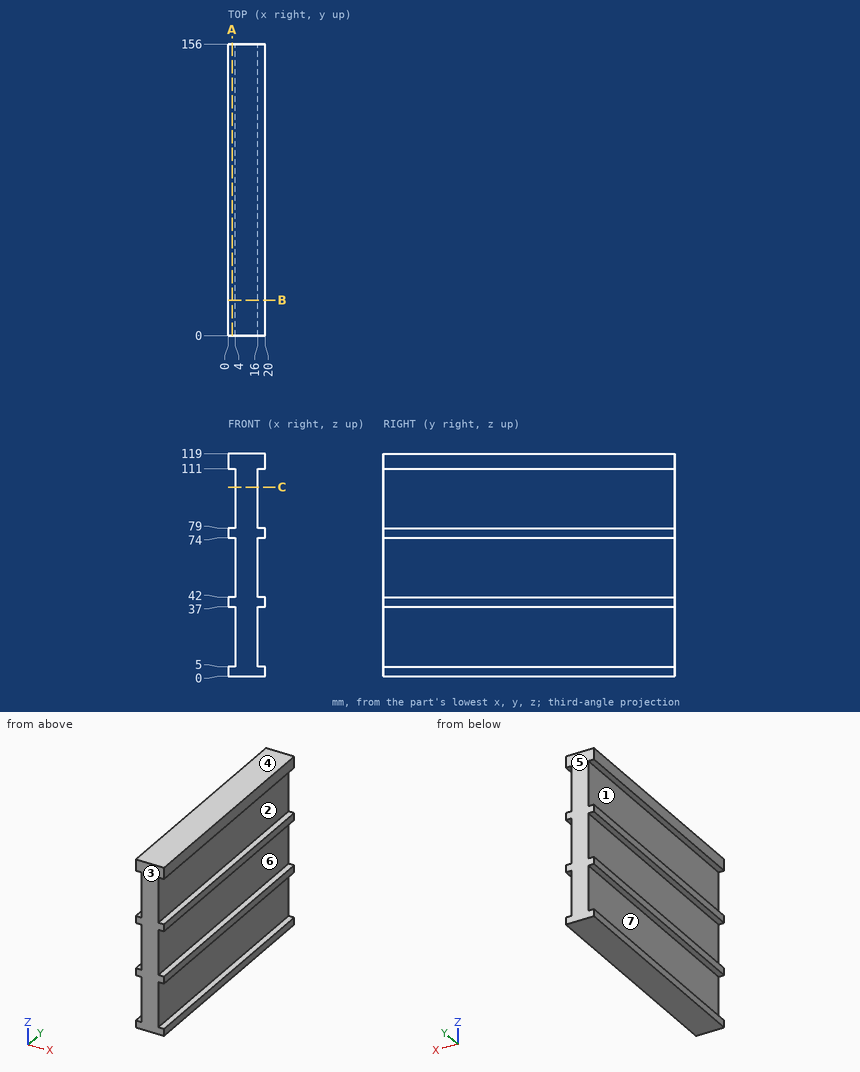
Source: three-view drawing plus pictorial views. Frame: mm from the lowest corner of the part. A direction names the side the tool comes from. Coordinates: 2 decimals unless noted, no trailing zeros. Write each loop counter-clockwise with the first axis right and the second up, starting at its lowest first coordinate (ties: lowest second). Pieces come first, ordered by that corner, then holes. Notation, with made-up numbers: (62.5, -24) -> (118.5, -24) arc R15 cw to (118.5, -20) -> close; hole circle Ø1 at (49, -24). An arc over 180 degrees is marked (long way). Answer as a JSON object with one key per item and string values.
1. Section C-C on z = 101. Return the cut outline in (x, y).
Result set:
{"outline": "(4, 0) -> (16, 0) -> (16, 156) -> (4, 156) -> close"}
2. Material intervals for line 1 (Z direction, x = 3.25, y = 39); line 2 (X direction, y = 57.5, z = 6.5), sorted ascending. Write a range as from..to.
Result set:
{"line 1": "z = 0..5, 37..42, 74..79, 111..119", "line 2": "x = 4..16"}
3. First-contact query: P1, Ø3, axis at x = 1, y = 90, coming from the -Z side; P2, Ø9.5, axis at y = 40.5, z = 25, coming from the +X side; P3, Ø1, axis at y = 79.5, z = 72.5, coming from the -X side. Flat tips, straight axial feed; report the tip coordinate or a pass-through.
Result set:
{"P1": "stops at z = 0", "P2": "stops at x = 16", "P3": "stops at x = 4"}
4. Section B-B on y = 19. Return the cut outline in (x, z), then the cut area to 3 significant figures.
Result set:
{"outline": "(0, 0) -> (20, 0) -> (20, 5) -> (16, 5) -> (16, 37) -> (20, 37) -> (20, 42) -> (16, 42) -> (16, 74) -> (20, 74) -> (20, 79) -> (16, 79) -> (16, 111) -> (20, 111) -> (20, 119) -> (0, 119) -> (0, 111) -> (4, 111) -> (4, 79) -> (0, 79) -> (0, 74) -> (4, 74) -> (4, 42) -> (0, 42) -> (0, 37) -> (4, 37) -> (4, 5) -> (0, 5) -> close", "area": "1,610 mm2"}
5. Section A-A on x = 2.25. Return the cut outline in (y, z), then the cut area to 3 significant figures.
Result set:
{"outline": "(0, 0) -> (156, 0) -> (156, 5) -> (0, 5) -> close; (0, 37) -> (156, 37) -> (156, 42) -> (0, 42) -> close; (0, 74) -> (156, 74) -> (156, 79) -> (0, 79) -> close; (0, 111) -> (156, 111) -> (156, 119) -> (0, 119) -> close", "area": "3,590 mm2"}
6. Access query for the marked faces 5, 6 and 7. Directions: +Z, -Z, +X, -X, +Y, -Y. A direction counts if a zero-diameter tool reaches every point of the face in a straight line with its end or side. Return the directions, or none.
Result set:
{"face 5": "+Z, -Z, +X, -X, +Y", "face 6": "+X, +Y, -Y", "face 7": "-X, +Y, -Y"}
7. Mould query, pull axis Z, two halves, no side actions, for the marked faces 1, 2, 3 and 4. Classes: released by +Z, released by -Z, zero draft, split by the parting line, or undercut.
Result set:
{"face 1": "undercut", "face 2": "undercut", "face 3": "zero draft", "face 4": "released by +Z"}
